Could you check a few things on this model? Use its own coordinates, in mm. A direction names the side the tool comes from. Coordinates: 2 decimals unless noted, no trailing zeros. Write each loop counter-clockwise with the first axis right and the second up, starting at its lowest first coordinate (ties: lowest second). Pieces come first, ordered by that corner, then holes.
Item 1: I want a section at D-D on x = 399. Please give me the cut outline in (y, z).
Item 2: I want a section at B-B on x = 159. Please give me the cut outline in (y, z).
Item 3: Thinking about a two-plate mould opening in Z: for faces 1 (the flat face through (0, 8, -237)), 2 (the cylindrical face through (408.168, 4.93, -57.532)), 3 (the cylindrical face through (397.68, 4.93, -430.71)), which applies, +Z half, -Z half, draft (parallel to the pull), parting line (faces both ways), or undercut?
Item 4: I want a section at A-A on z = -204. Please give me the cut outline in (x, y), then the cut area to 3 significant figures.
Item 5: If I drill on probe 1 along X at (y, z) = (9, -395); probe 2 along X at (y, z) = (4.5, -233.5); probe 3 along Z at (x, y) = (362.5, 4.5), over which ranges is the centre line in solid material (lowest first)?
Item 6: Which directions (+Z, -Z, +X, -X, +Y, -Y) give clear straight access to the entire face, cutting with the end or side of a thin tool? Please do faces 4 (the flat face through (436, 8, -230)), 5 (the cylindrical face through (398.16, 4.93, -67.32)), 6 (the cylindrical face through (236.43, 8.11, -219.82)).
Item 7: I want a section at C-C on z = -121.5. Please give me the cut outline in (x, y).
Autodesk Inventor part; units mm, degrees
ref_plane "YZ Plane" through (0, 0, 0) normal (1, 0, 0) x (0, 1, 0)
ref_plane "XZ Plane" through (0, 0, 0) normal (0, 1, 0) x (-1, 0, 0)
ref_plane "XY Plane" through (0, 0, 0) normal (0, 0, 1) x (1, 0, 0)
sketch "Sketch1" plane through (0, 0, 0) normal (0, 1, 0) x (-1, 0, 0)
  line L0 (0, 0) -> (-436, 0)
  line L1 (-436, 0) -> (-436, -467)
  line L2 (-436, -467) -> (0, -467)
  line L3 (0, -467) -> (0, 0)
  dimension "d0" = 436
  dimension "d1" = 467
extrude "Extrusion1" add sketch "Sketch1" along normal blind 16
sketch "Sketch2" plane through (0, 16, 0) normal (0, 1, 0) x (1, 0, 0)
  circle A0 centre (366, 459.5) radius 2
  line L0 (436, 467) -> (0, 467)
  circle A1 centre (336, 459.5) radius 2
  circle A2 centre (100, 459.5) radius 2
  circle A3 centre (70, 459.5) radius 2
  line L1 (436, 0) -> (436, 467)
  line L2 (0, 467) -> (0, 0)
  circle A4 centre (218, 233.5) radius 4.5
  circle A5 centre (118, 131.05) radius 2
  circle A6 centre (318, 131.05) radius 2
  circle A7 centre (118, 367.05) radius 2
  circle A8 centre (318, 367.05) radius 2
  line L3 (0, 0) -> (436, 0)
  line L4 (218, 218.5) -> (218, 165.5)
  line L5 (218, 233.5) -> (338, 233.5) construction
  arc A9 (266, 185.5) -> (246.243, 209.1616) centre (218, 165.5) ccw
  line L6 (266, 185.5) -> (302.8528, 148.6472)
  circle A10 centre (218, 233.5) radius 120
  line L7 (231.5946, 239.8393) -> (326.7569, 284.2142)
  circle A11 centre (218, 233.5) radius 15
  arc A12 (326.7569, 284.2142) -> (231.5946, 239.8393) centre (279.1758, 262.0267) ccw
  arc A13 (233, 233.5) -> (246.243, 209.1616) centre (261.9865, 233.5) ccw
  arc A14 (296.9937, 154.5063) -> (308.697, 154.9248) centre (302.6505, 160.1632) ccw
  point P0 (228.6066, 222.8934)
  dimension "d4" = 4
  dimension "d9" = 30
  dimension "d18" = 7.5
  dimension "d24" = 30
  dimension "d31" = 70
  dimension "d32" = 70
  dimension "d33" = 9
  dimension "d34" = 218
  dimension "d35" = 233.5
  dimension "d36" = 4
  dimension "d37" = 102.45
  dimension "d40" = 200
  dimension "d43" = 236
  dimension "d47" = 100
  dimension "d58" = 68
  dimension "d59" = 90
  dimension "d63" = 52
  dimension "d64" = 240
  dimension "d66" = 115
  dimension "d67" = 30
  dimension "d68" = 105
  dimension "d69" = 45
  dimension "d70" = 8
  dimension "d98" = 7.5
extrude "Extrusion2" cut sketch "Sketch2" against normal through all contours A0 | A1 | A3 | A4 | A5 | A6 | A7 | A8 | A9 A13 A11 L7 A10 A14 L6 | A12 L7
sketch "Sketch3" plane through (0, 0, 0) normal (0, -1, 0) x (1, 0, 0)
  circle A0 centre (218, -165.5) radius 52
  circle A1 centre (218, -233.5) radius 4.5
  arc A2 (246.243, -209.1616) -> (266, -185.5) centre (218, -165.5) ccw
  line L0 (233, -195.5) -> (138, -195.5)
  line L1 (128, -185.5) -> (128, -145.5)
  line L2 (138, -135.5) -> (233, -135.5)
  line L3 (243, -145.5) -> (243, -185.5)
  arc A3 (138, -135.5) -> (128, -145.5) centre (138, -145.5) ccw
  arc A4 (128, -185.5) -> (138, -195.5) centre (138, -185.5) ccw
  arc A5 (233, -195.5) -> (243, -185.5) centre (233, -185.5) ccw
  arc A6 (243, -145.5) -> (233, -135.5) centre (233, -145.5) ccw
  point P0 (0, 0)
  point P1 (243, -195.5)
  point P2 (128, -135.5)
  point P3 (128, -195.5)
  point P4 (243, -135.5)
  dimension "d71" = 104
  dimension "d73" = 115
  dimension "d74" = 60
  dimension "d75" = 30
  dimension "d76" = 25
  dimension "d97" = 10
extrude "Extrusion3" cut sketch "Sketch3" against normal blind 13 contours L0 A4 L1 A3 L2 A0 | A0 L2 A6 L3 A5 L0 picked at (210.7335, -163.9792)
sketch "Sketch4" plane through (0, 13, 0) normal (0, -1, 0) x (1, 0, 0)
  line L0 (134.5, -165.5) -> (134.5, -190.5)
  line L1 (130.5, -190.5) -> (130.5, -165.5)
  arc A0 (130.5, -190.5) -> (134.5, -190.5) centre (132.5, -190.5) ccw
  arc A1 (134.5, -165.5) -> (130.5, -165.5) centre (132.5, -165.5) ccw
  line L2 (233, -195.5) -> (138, -195.5)
  line L3 (128, -185.5) -> (128, -145.5)
  circle A2 centre (148, -140.5) radius 1.75
  line L4 (138, -135.5) -> (233, -135.5)
  circle A3 centre (233, -140.5) radius 1.75
  circle A4 centre (148, -190.5) radius 1.75
  circle A5 centre (233, -190.5) radius 1.75
  point P0 (0, 0)
  point P1 (243, -195.5)
  point P2 (128, -195.5)
  point P3 (128, -135.5)
  point P4 (243, -135.5)
  dimension "d79" = 4
  dimension "d81" = 25
  dimension "d82" = 5
  dimension "d83" = 2.5
  dimension "d84" = 3.5
  dimension "d85" = 5
  dimension "d86" = 20
  dimension "d89" = 85
  dimension "d92" = 50
extrude "Extrusion4" cut sketch "Sketch4" against normal through all
sketch "Sketch5" plane through (0, 16, 0) normal (0, 1, 0) x (1, 0, 0)
  circle A0 centre (100, 459.5) radius 2
  circle A1 centre (70, 459.5) radius 2
  point P0 (0, 0)
  dimension "d99" = 0
  dimension "d100" = 30
extrude "Extrusion5" cut sketch "Sketch5" against normal through all contours A0
sketch "Sketch6" plane through (0, 0, 0) normal (0, -1, 0) x (1, 0, 0)
  line L0 (376, -453.55) -> (60, -453.55)
  line L1 (15, -408.55) -> (15, -89)
  line L2 (60, -44) -> (376, -44)
  line L3 (421, -89) -> (421, -408.55)
  line L4 (0, -467) -> (0, 0)
  line L5 (436, 0) -> (436, -467)
  line L6 (0, 0) -> (436, 0)
  line L7 (436, -467) -> (0, -467)
  arc A0 (15, -408.55) -> (60, -453.55) centre (60, -408.55) ccw
  arc A1 (376, -453.55) -> (421, -408.55) centre (376, -408.55) ccw
  arc A2 (421, -89) -> (376, -44) centre (376, -89) ccw
  arc A3 (60, -44) -> (15, -89) centre (60, -89) ccw
  line L8 (60, -439.55) -> (376, -439.55)
  arc A4 (376, -439.55) -> (407, -408.55) centre (376, -408.55) ccw
  line L9 (407, -408.55) -> (407, -89)
  arc A5 (407, -89) -> (376, -58) centre (376, -89) ccw
  line L10 (376, -58) -> (60, -58)
  arc A6 (60, -58) -> (29, -89) centre (60, -89) ccw
  line L11 (29, -89) -> (29, -408.55)
  arc A7 (29, -408.55) -> (60, -439.55) centre (60, -408.55) ccw
  dimension "d104" = 15
  dimension "d105" = 15
  dimension "d106" = 44
  dimension "d107" = 13.45
  dimension "d108" = 45
  dimension "d109" = 14
extrude "Extrusion6" cut sketch "Sketch6" against normal blind 10 contours L0 A0 L1 A3 L2 A2 L3 A1
equation "\"d36\" = screws"
properties part number "bin_lid"
Response values:
1. outline: (0, -467) - (16, -467) - (16, 0) - (0, 0) - (0, -50.32) - (10, -50.32) - (10, -68.22) - (0, -68.22) - (0, -429.33) - (10, -429.33) - (10, -447.23) - (0, -447.23) - close
2. outline: (0, -467) - (16, -467) - (16, 0) - (0, 0) - (0, -44) - (10, -44) - (10, -58) - (0, -58) - (0, -135.5) - (13, -135.5) - (13, -195.5) - (0, -195.5) - (0, -439.55) - (10, -439.55) - (10, -453.55) - (0, -453.55) - close
3. face 1: draft
3. face 2: undercut
3. face 3: undercut
4. outline: (0, 0) - (15, 0) - (15, 10) - (29, 10) - (29, 0) - (252.95, 0) - (252.95, 16) - (0, 16) - close; (334.32, 0) - (407, 0) - (407, 10) - (421, 10) - (421, 0) - (436, 0) - (436, 16) - (334.32, 16) - close
4. area: 5,390 mm2
5. probe 1: x = 0 to 15, 29 to 407, 421 to 436
5. probe 2: x = 0 to 15, 29 to 213.5, 222.5 to 233, 338 to 407, 421 to 436
5. probe 3: z = -467 to -453.55, -439.55 to -58, -44 to 0
6. face 4: +Z, -Z, +X, +Y, -Y
6. face 5: -Y
6. face 6: +Y, -Y
7. outline: (0, 0) - (15, 0) - (15, 10) - (29, 10) - (29, 0) - (407, 0) - (407, 10) - (421, 10) - (421, 0) - (436, 0) - (436, 16) - (0, 16) - close
